Model file for the job. Use its own axes, mm. A direction names the side the tool comes from. Round coordinates to 2 decimals unless told otherwise and drop trailing zeros. Order: outer loops, then holes, each group sorted by start corner. A loop starts at its lowest first (then second) coordinate and runs counter-clockwise, first axis right, second up. Notation, with made-up numbers: (52.5, 78.25) - (109.5, 78.25) arc R12 ccw to (109.5, 95.25) - close; hole circle Ø3 at (27, -25.75). An arc over 180 degrees is marked (long way). Answer as CSV lines item,"result". Start each with the question number.
1. Band-saw the part on B-B on z = 0. List the corners of the cut face in (x, y) (3 decimals), then the cut area to 3 significant figures.
2. Band-saw the part on D-D on y = -0.5. List the corners of the cut face in (x, z), then the cut area to 3 significant figures.
3. Pull direction Y, two halves, no side cores. Call faces 1 (the face through (4.7, -12.734, 3.3)), 2 (the face through (8, -20.36, 4)), 3 (the face through (1.162, -8.957, -1.076)), 4 (the face through (2, -5.284, -3)): released by +Y, released by -Y, zero draft, split by the parting line, or undercut.
4. Wall check: line 1 along X through (y, z) = (-4.5, 0); line 2 along X through (y, z) = (-7, 0); line 3 along Z through (x, y) = (9.75, -1). Give the ranges that are in metal, low to high. Write a range as [from, to].
5. Band-saw the part on A-A on y = -10.25. List the corners of the cut face in (x, z).
6. Band-saw the part on C-C on x = 12.75. List the corners of the cut face in (y, z).
7. Pin check, flat tips, straight feed: pin 1 Ø1.5 at (y, z) = (-3.5, 3) entering from -X; pin 2 Ø1 at (x, z) = (2.5, -3) entering from -Y; pin 3 Ø1 at (x, y) = (6.5, 1) entering from +Z; pin 4 Ø4 at (x, z) = (7.81, 0) entering from -Y. Stop position of each tip, or through.
8. 3-axis set-ups, long thin cutter, end or side, ignore diameter. For faces 5 (the face through (10.2, -9, 6.3)), 6 (the face through (13.928, -0.599, -0.269)), 7 (the face through (3.666, -12.899, -1.306)): which of +Z, -Z, +X, -X, +Y, -Y reach the whole face in a straight line?
```python
from build123d import *

# Parameters (mm, degrees)
CROQUIS1_W            = 2.662106529
CROQUIS1_H            = 9.24
CORTAR_EXTRUIR1_REACH = 25.043


with BuildPart() as part:
    # Croquis1 → Revolución1 (revolve)
    with BuildSketch(Plane.XY):
        with Locations((3.024759969, -0.663755178)):
            Rectangle(CROQUIS1_W, CROQUIS1_H)
        Polygon((4.355813233, -12.733755178), (4.355813233, -5.283755178), (1.693706704, -5.283755178), (0.033706704, -5.283755178), (0.033706704, -12.733755178), (3.465, -12.733755178), align=None)
        Polygon((4.355813233, -13.950813233), (4.355813233, -12.733755178), (3.465, -12.733755178), (3.465, -13.06), align=None)
        with BuildLine():
            Line((4.355813233, -14.607729599), (4.355813233, -13.950813233))
            Line((4.355813233, -13.950813233), (3.465, -13.06))
            Line((3.465, -13.06), (3.465, -16.464646325))
            ThreePointArc((3.465, -16.464646325), (3.80150201, -15.483943474), (4.355813233, -14.607729599))
        make_face()
        with BuildLine():
            Line((3.465, -16.464646325), (3.465, -13.06))
            ThreePointArc((3.465, -13.06), (1.725988008, -16.53567688), (2.418118888, -20.36))
            Line((2.418118888, -20.36), (3.465, -20.36))
            Line((3.465, -20.36), (3.465, -18.352767084))
            ThreePointArc((3.465, -18.352767084), (3.363706704, -17.408706704), (3.465, -16.464646325))
        make_face()
        with BuildLine():
            Line((3.465, -20.36), (4.355813233, -20.36))
            Line((4.355813233, -20.36), (3.909582187, -19.544195349))
            ThreePointArc((3.909582187, -19.544195349), (3.644512403, -18.964444111), (3.465, -18.352767084))
            Line((3.465, -18.352767084), (3.465, -20.36))
        make_face()
    revolve(axis=Axis((7.813706704, 3.956244822, 0), (0, -1, 0)))

    # Croquis2 → Cortar-Extruir1 (cut, up to next)
    with BuildSketch(Plane(origin=(0, -5.283755178, 0), x_dir=(-1, 0, 0), z_dir=(0, 1, 0)), mode=Mode.PRIVATE) as cortar_extruir1_sk1:
        with BuildLine():
            ThreePointArc((-6.509101958, 7.669837447), (-10.518804576, 7.294576445), (-13.803678403, 4.964739575))
            Line((-13.803678403, 4.964739575), (-6.509101958, 7.669837447))
        make_face()
    cortar_extruir1_tool1 = extrude(cortar_extruir1_sk1.sketch, amount=-CORTAR_EXTRUIR1_REACH, mode=Mode.PRIVATE) & part.part
    # Croquis2 → Cortar-Extruir1 (cut, up to next)
    with BuildSketch(Plane(origin=(0, -5.283755178, 0), x_dir=(-1, 0, 0), z_dir=(0, 1, 0)), mode=Mode.PRIVATE) as cortar_extruir1_sk2:
        with BuildLine():
            Line((-15.108283149, -2.705097871), (-13.803678403, 4.964739575))
            ThreePointArc((-13.803678403, 4.964739575), (-15.483544151, 1.304604746), (-15.108283149, -2.705097871))
        make_face()
    cortar_extruir1_tool2 = extrude(cortar_extruir1_sk2.sketch, amount=-CORTAR_EXTRUIR1_REACH, mode=Mode.PRIVATE) & part.part
    # Croquis2 → Cortar-Extruir1 (cut, up to next)
    with BuildSketch(Plane(origin=(0, -5.283755178, 0), x_dir=(-1, 0, 0), z_dir=(0, 1, 0)), mode=Mode.PRIVATE) as cortar_extruir1_sk3:
        with BuildLine():
            Line((-9.11831145, -7.669837447), (-15.108283149, -2.705097871))
            ThreePointArc((-15.108283149, -2.705097871), (-12.77844628, -5.989971699), (-9.11831145, -7.669837447))
        make_face()
    cortar_extruir1_tool3 = extrude(cortar_extruir1_sk3.sketch, amount=-CORTAR_EXTRUIR1_REACH, mode=Mode.PRIVATE) & part.part
    # Croquis2 → Cortar-Extruir1 (cut, up to next)
    with BuildSketch(Plane(origin=(0, -5.283755178, 0), x_dir=(-1, 0, 0), z_dir=(0, 1, 0)), mode=Mode.PRIVATE) as cortar_extruir1_sk4:
        with BuildLine():
            Line((-1.823735006, -4.964739575), (-9.11831145, -7.669837447))
            ThreePointArc((-9.11831145, -7.669837447), (-5.108608833, -7.294576445), (-1.823735006, -4.964739575))
        make_face()
    cortar_extruir1_tool4 = extrude(cortar_extruir1_sk4.sketch, amount=-CORTAR_EXTRUIR1_REACH, mode=Mode.PRIVATE) & part.part
    # Croquis2 → Cortar-Extruir1 (cut, up to next)
    with BuildSketch(Plane(origin=(0, -5.283755178, 0), x_dir=(-1, 0, 0), z_dir=(0, 1, 0)), mode=Mode.PRIVATE) as cortar_extruir1_sk5:
        with BuildLine():
            ThreePointArc((-0.033706704, 0), (-0.156024133, 1.374153423), (-0.51913026, 2.705097871))
            Line((-0.51913026, 2.705097871), (-1.823735006, -4.964739575))
            ThreePointArc((-1.823735006, -4.964739575), (-0.494882351, -2.638789513), (-0.033706704, 0))
        make_face()
    cortar_extruir1_tool5 = extrude(cortar_extruir1_sk5.sketch, amount=-CORTAR_EXTRUIR1_REACH, mode=Mode.PRIVATE) & part.part
    # Croquis2 → Cortar-Extruir1 (cut, up to next)
    with BuildSketch(Plane(origin=(0, -5.283755178, 0), x_dir=(-1, 0, 0), z_dir=(0, 1, 0)), mode=Mode.PRIVATE) as cortar_extruir1_sk6:
        with BuildLine():
            ThreePointArc((-0.51913026, 2.705097871), (-2.848967129, 5.989971699), (-6.509101958, 7.669837447))
            Line((-6.509101958, 7.669837447), (-0.51913026, 2.705097871))
        make_face()
    cortar_extruir1_tool6 = extrude(cortar_extruir1_sk6.sketch, amount=-CORTAR_EXTRUIR1_REACH, mode=Mode.PRIVATE) & part.part
    add(cortar_extruir1_tool1.solids().sort_by_distance((10.302222, -5.283755, 6.710539))[0], mode=Mode.SUBTRACT)
    add(cortar_extruir1_tool2.solids().sort_by_distance((14.869461, -5.283755, 1.200152))[0], mode=Mode.SUBTRACT)
    add(cortar_extruir1_tool3.solids().sort_by_distance((12.380946, -5.283755, -5.510387))[0], mode=Mode.SUBTRACT)
    add(cortar_extruir1_tool4.solids().sort_by_distance((5.325191, -5.283755, -6.710539))[0], mode=Mode.SUBTRACT)
    add(cortar_extruir1_tool5.solids().sort_by_distance((0.757952, -5.283755, -1.200152))[0], mode=Mode.SUBTRACT)
    add(cortar_extruir1_tool6.solids().sort_by_distance((3.246467, -5.283755, 5.510387))[0], mode=Mode.SUBTRACT)


solid = part.part
```
Reply:
1,outline,"(0.979, -12.734) - (3.465, -12.734) - (3.465, -13.06) arc R6.15 ccw to (2.418, -20.36) - (4.356, -20.36) - (3.91, -19.544) arc R4.45 cw to (4.356, -14.608) - (4.356, 3.956) - (1.694, 3.956) - (1.694, -5.284) - (0.979, -5.284) - close; (11.272, -20.36) - (13.209, -20.36) arc R6.15 ccw to (12.162, -13.06) - (12.162, -12.734) - (14.648, -12.734) - (14.648, -5.284) - (13.934, -5.284) - (13.934, 3.956) - (11.272, 3.956) - (11.272, -14.608) arc R4.45 cw to (11.718, -19.544) - close"
1,area,"125 mm2"
2,outline,"circle Ø12.24 at (7.81, 0); hole circle Ø6.92 at (7.81, 0)"
2,area,"80.1 mm2"
3,face 1,"undercut"
3,face 2,"released by -Y"
3,face 3,"zero draft"
3,face 4,"released by +Y"
4,line 1,"x = [1.69, 4.36], [11.27, 13.93]"
4,line 2,"x = [0.98, 4.36], [11.27, 14.65]"
4,line 3,"z = [-5.81, -2.86], [2.86, 5.81]"
5,outline,"(0.52, 2.71) - (1.82, -4.96) - (9.12, -7.67) - (15.11, -2.71) - (13.8, 4.96) - (6.51, 7.67) - close; hole circle Ø6.92 at (7.81, 0)"
6,outline,"(-20.36, -2.18) arc R3.67 ccw (long way) to (-20.36, 2.18) - close; (-12.73, -4.66) - (-5.28, -4.66) - (-5.28, -3.62) - (3.96, -3.62) - (3.96, 3.62) - (-5.28, 3.62) - (-5.28, 5.36) - (-12.73, 5.36) - close"
7,pin 1,"stops at x = 2.12"
7,pin 2,"stops at y = -19.95"
7,pin 3,"stops at z = 6.07"
7,pin 4,"passes through"
8,face 5,"+Z, +X, +Y, -Y"
8,face 6,"+Y"
8,face 7,"none"
